For this review, take the finished solid that the model builds, in its own axes (mm). A direction names the side the tool comes from. Coordinates: 2 decimals unless noted, no trailing zeros. Write each loop counter-clockwise with the first axis right and the second up, starting at its lowest first coordinate (ties: lowest second). Pieces come first, ordered by that corner, then holes. Notation, with made-up numbers: (52.25, -8) - (68.25, -8) arc R30 ccw to (68.25, 16) - close; hole circle Ø7 at (75, -28). An arc over 180 degrees is marked (long way). Use one line per item in the form item = value. Start each with the question number.
1) We need section A-A (z = 17.25). Give the boundary of the cut face in (x, y).
2) We need section D-D (y = -27.5). Give the boundary of the cut face in (x, z), plus the area to 3 significant figures.
3) Insertion check: P1, Ø16, axis at x = -24.85, y = -38.68, coming from the -Z side; P2, Ø2, axis at x = -31.5, z = 18.5, coming from the +Y side; P3, Ø6, axis at x = -9.5, y = -23.5, coming from the +Z side; P4, Ø7, axis at y = -34.5, z = 34.5, coming from the +X side. Each pin has a flat end and moves straight along its axis. Give the tip position at first contact, or say it passes through.
4) We need section B-B (x = -22). Give the boundary of the cut face in (y, z).
5) Mouldability with a two-part tool opening along Y and no side actions: class faces 1 (the cylindrical face through (-29.85, -12.44, 30.13)), 2 (the cylindrical face through (-24.203, -33.727, 30.131)), 3 (the flat face through (-25, 0, 26)), 4 (the flat face through (-3.255, -25, 23)) as pulls with the +Y half, pulls with the -Y half, needs draft (parallel to the pull), parting line crosses it, or undercut.
6) Tool access review of faces 5 (the flat face through (-34.283, -25, 34)), 6 (the flat face through (-14.968, -25, 33)), 7 (the flat face through (-14.968, -25, 20)), 8 (the flat face through (-25, -50, 26)): name each direction out of +Z, -Z, +X, -X, +Y, -Y from which nothing blocks a thin tool from reaching the whole face with its end or side.
7) We need section C-C (y = -39.5). Give the boundary of the cut face in (x, z), plus the area to 3 significant figures.
8) For L1, parallel to X at y = -38.5, z = 22; L2, parallel to Y at x = -23.5, z = 27; L3, parallel to Y at x = -24.5, z = 26, list the stretches that pass through material, from the lowest coordinate up. Write a range as from..to.
```python
from build123d import *

# Parameters (mm, degrees)
F1_DEPTH = 50
F3_D     = 10
F4_D     = 10


with BuildPart() as f1:
    # F0 (on Front) → F1 (new body)
    with BuildSketch(Plane.XZ):
        Polygon((-45.584108, 30.324244), (-45.584108, 15.324244), (-34.282739, 15.324244), (-34.282739, 23.748901), (-14.967671, 23.748901), (-14.967671, 15.324244), (-3.255342, 15.324244), (-3.255342, 30.324244), (-14.967671, 30.324244), (-14.967671, 36.694106), (-34.282739, 36.694106), (-34.282739, 30.324244), align=None)
    extrude(amount=F1_DEPTH)

    # F3 (through all)
    with Locations(Plane.XY.offset(36.694106)):
        with Locations((-25.230138, -10.524154)):
            Hole(F3_D / 2)

    # F4 (through all)
    with Locations(Plane.XY.offset(36.694106)):
        with Locations((-24.854114, -38.68451)):
            Hole(F4_D / 2)


solid = f1.part
```
Determined:
q1.outline = (-45.58, -50) - (-34.28, -50) - (-34.28, 0) - (-45.58, 0) - close; (-14.97, -50) - (-3.26, -50) - (-3.26, 0) - (-14.97, 0) - close
q2.outline = (-45.58, 15.32) - (-34.28, 15.32) - (-34.28, 23.75) - (-14.97, 23.75) - (-14.97, 15.32) - (-3.26, 15.32) - (-3.26, 30.32) - (-14.97, 30.32) - (-14.97, 36.69) - (-34.28, 36.69) - (-34.28, 30.32) - (-45.58, 30.32) - close
q2.area = 595 mm²
q3.P1 = 23.75
q3.P2 = through
q3.P3 = 30.32
q3.P4 = -14.97
q4.outline = (-50, 23.75) - (-42.79, 23.75) - (-42.79, 36.69) - (-50, 36.69) - close; (-34.58, 23.75) - (-14.34, 23.75) - (-14.34, 36.69) - (-34.58, 36.69) - close; (-6.71, 23.75) - (0, 23.75) - (0, 36.69) - (-6.71, 36.69) - close
q5.face_1 = undercut
q5.face_2 = undercut
q5.face_3 = pulls with the +Y half
q5.face_4 = needs draft
q6.face_5 = +Z, -X, +Y, -Y
q6.face_6 = +Z, +X, +Y, -Y
q6.face_7 = -Z, +Y, -Y
q6.face_8 = +Z, -Z, +X, -X, -Y
q7.outline = (-45.58, 15.32) - (-34.28, 15.32) - (-34.28, 23.75) - (-29.79, 23.75) - (-29.79, 36.69) - (-34.28, 36.69) - (-34.28, 30.32) - (-45.58, 30.32) - close; (-19.92, 23.75) - (-14.97, 23.75) - (-14.97, 15.32) - (-3.26, 15.32) - (-3.26, 30.32) - (-14.97, 30.32) - (-14.97, 36.69) - (-19.92, 36.69) - close
q7.area = 468 mm²
q8.L1 = -45.58..-34.28, -14.97..-3.26
q8.L2 = -50..-43.5, -33.87..-15.22, -5.83..0
q8.L3 = -50..-43.67, -33.7..-15.47, -5.58..0
